from build123d import *

# Parameters (mm, degrees)
F0_W     = 71.12
F0_H     = 53.34
F0_W_2   = 101.6
F0_H_2   = 76.2
F1_DEPTH = 3.175
F2_DEPTH = 15.875


with BuildPart() as f1:
    # F0 (on Top) → F1 (new body)
    with BuildSketch(Plane.XY):
        Rectangle(F0_W, F0_H)
        Rectangle(F0_W_2, F0_H_2)
        Rectangle(F0_W, F0_H, mode=Mode.SUBTRACT)
    extrude(amount=F1_DEPTH)

    # F0 (on Top) → F2 (join)
    with BuildSketch(Plane.XY):
        Rectangle(F0_W, F0_H)
    extrude(amount=F2_DEPTH)


solid = f1.part
Geometry check sheet. Reference: the model listing, model coordinates, mm. A direction names the side the tool comes from. Give positions to 0.01 mm unless a question says otherwise; leave off trailing zeros. Write each loop counter-clockwise with the first axis right and the second up, starting at its lowest first coordinate (ties: lowest second). Pieces come first, ordered by that corner, then holes. Notation, with made-up numbers: M -9.75,33.25 L 22.25,33.25 A27 ccw 22.25,58.25 Z; hole C 37.25,-15 d1. An arc over 180 degrees is marked long. Answer as CSV lines item,"result". Start each with the question number.
Q1. Section check A-A, the plane y = -25. Record the cut outline in (x, z) (3 decimals), then the cut area to 3 significant figures.
Q2. Material ranges on L1, parallel to X at y = 19, z = 8; L2, parallel to Z at x = -36.5, y = -18 (3 decimals); L3, parallel to Y at x = 3, z = 15, recorded low to high.
Q3. Section check B-B, the plane x = 16.5. Record the cut outline in (y, z) (3 decimals), then the cut area to 3 significant figures.
Q4. Tool access check on faces 1 (the face through (-1, -38.1, 2)), 2 (the face through (-35.56, 0, 9)), 3 (the face through (0, -26.67, 9)), 4 (the face through (35.56, 0, 9)), 5 (the face through (0, 26.67, 9)). Record the directions out of +Z, -Z, +X, -X, +Y, -Y that give a thin tool (end or side, any length) a straight path to the whole face; none if there is none.
Q5. Section check C-C, the plane z = 10.75. Record the cut outline in (x, y), then the cut area to 3 significant figures.
Q6. Go/stop test with flat-tipped pins: pin 1 (4 mm diameter, centred on y = 10.5, z = 9.5, fed in from -X); pin 2 (8 mm diameter, centred on x = -13.5, z = 6, fed in from +Y); pin 3 (1 mm diameter, centred on x = -11, z = 11.5, fed in from -Y). Record where each tip stops, or that it passes through.
Q7. Section check D-D, the plane y = 31. Record the cut outline in (x, z) (3 decimals), then the cut area to 3 significant figures.
Geometry says:
1,outline,"M -50.8,0 L 50.8,0 L 50.8,3.175 L 35.56,3.175 L 35.56,15.875 L -35.56,15.875 L -35.56,3.175 L -50.8,3.175 Z"
1,area,"1,230 mm^2"
2,L1,"-35.56 to 35.56"
2,L2,"0 to 3.175"
2,L3,"-26.67 to 26.67"
3,outline,"M -38.1,0 L 38.1,0 L 38.1,3.175 L 26.67,3.175 L 26.67,15.875 L -26.67,15.875 L -26.67,3.175 L -38.1,3.175 Z"
3,area,"919 mm^2"
4,face 1,"+Z, -Z, +X, -X, -Y"
4,face 2,"+Z, -X, +Y, -Y"
4,face 3,"+Z, +X, -X, -Y"
4,face 4,"+Z, +X, +Y, -Y"
4,face 5,"+Z, +X, -X, +Y"
5,outline,"M -35.56,-26.67 L 35.56,-26.67 L 35.56,26.67 L -35.56,26.67 Z"
5,area,"3,790 mm^2"
6,pin 1,"x = -35.56"
6,pin 2,"y = 38.1"
6,pin 3,"y = -26.67"
7,outline,"M -50.8,0 L 50.8,0 L 50.8,3.175 L -50.8,3.175 Z"
7,area,"323 mm^2"
